from build123d import *

# Parameters (mm, degrees)
SKETCH_1_R      = 6.25
EXTRUDE_1_DEPTH = 15
SKETCH_2_W      = 27
SKETCH_2_H      = 18
EXTRUDE_2_DEPTH = 3
EXTRUDE_START   = 13.5
SKETCH_3_R      = 1.65
EXTRUDE_3_DEPTH = 5
EXTRUDE_START_2 = -13.5
SKETCH_3_2_R    = 1.65
EXTRUDE_4_DEPTH = 5
EXTRUDE_5_DEPTH = 5
SKETCH_5_R      = 2.5
EXTRUDE_6_DEPTH = 5


with BuildPart() as part:
    # ｽｹｯﾁ1 → ﾎﾞｽ - 押し出し1 (new body)
    with BuildSketch(Plane.XY):
        Circle(SKETCH_1_R)
    extrude(amount=EXTRUDE_1_DEPTH)

    # ｽｹｯﾁ2 → ﾎﾞｽ - 押し出し2 (add)
    with BuildSketch(Plane.XY.offset(15)):
        Rectangle(SKETCH_2_W, SKETCH_2_H)
    extrude(amount=EXTRUDE_2_DEPTH)

    # ｽｹｯﾁ3 → ﾎﾞｽ - 押し出し3 (add)
    with BuildSketch(Plane(origin=(0, 0, 0), x_dir=(0, 0, -1), z_dir=(1, 0, 0)).offset(EXTRUDE_START)):
        with BuildLine():
            Line((-18, 9), (-29.724032154, 4.69336906))
            ThreePointArc((-29.724032154, 4.69336906), (-33, 0), (-29.724032154, -4.69336906))
            Line((-29.724032154, -4.69336906), (-18, -9))
            Line((-18, -9), (-18, 9))
        make_face()
        with Locations((-28, 0)):
            Circle(SKETCH_3_R, mode=Mode.SUBTRACT)
    extrude(amount=-EXTRUDE_3_DEPTH)

    # ｽｹｯﾁ3<2> → ﾎﾞｽ - 押し出し4 (add)
    with BuildSketch(Plane(origin=(0, 0, 0), x_dir=(0, 0, -1), z_dir=(1, 0, 0)).offset(EXTRUDE_START_2)):
        with BuildLine():
            Line((-18, 9), (-29.724032154, 4.69336906))
            ThreePointArc((-29.724032154, 4.69336906), (-33, 0), (-29.724032154, -4.69336906))
            Line((-29.724032154, -4.69336906), (-18, -9))
            Line((-18, -9), (-18, 9))
        make_face()
        with Locations((-28, 0)):
            Circle(SKETCH_3_2_R, mode=Mode.SUBTRACT)
    extrude(amount=EXTRUDE_4_DEPTH)

    # ｽｹｯﾁ4 → ﾎﾞｽ - 押し出し5 (add, symmetric)
    with BuildSketch(Plane(origin=(0, 0, 0), x_dir=(1, 0, 0), z_dir=(0, 1, 0))):
        with BuildLine():
            Line((-13.5, -63), (-13.5, -3))
            ThreePointArc((-13.5, -3), (-43.5, -33), (-13.5, -63))
        make_face()
    extrude(amount=EXTRUDE_5_DEPTH, both=True)

    # ｽｹｯﾁ5 → ﾎﾞｽ - 押し出し6 (add)
    with BuildSketch(Plane.XY.offset(40)):
        with BuildLine():
            Line((-30, 5), (-30, 10))
            ThreePointArc((-30, 10), (-25, 15), (-20, 10))
            Line((-20, 10), (-20, 5))
            Line((-20, 5), (-30, 5))
        make_face()
        with Locations((-25, 10)):
            Circle(SKETCH_5_R, mode=Mode.SUBTRACT)
    extrude_6 = extrude(amount=EXTRUDE_6_DEPTH)

    # ﾐﾗｰ1: ﾎﾞｽ - 押し出し6 across plane
    add(extrude_6.mirror(Plane.ZX))


solid = part.part
Part model, mm, in its own coordinate system. A direction names the side the tool comes from. Give positions to 0.01 mm unless a question says otherwise; leave off trailing zeros. Loops run counter-clockwise (first coordinate to the right, second up) from the corner with the lowest first, then second, coordinate; pieces in that order, holes last.
(1) Pull direction X, two halves, no side cores. Call faces 6 (the cylindrical face through (-11.04, 0.07, 29.65)), 7 (the cylindrical face through (-25, 15, 42)), 8 (the cylindrical face through (-27, 8.5, 42.5)), 9 (the cylindrical face through (-27, -8.5, 42.5)): pulls with the +X half, pulls with the -X half, needs draft (parallel to the pull), parting line crosses it, or undercut.
Return value:
face 6: needs draft
face 7: parting line crosses it
face 8: undercut
face 9: undercut
(2) Band-saw the part on A-A (x = -10.5). Write the cut outline in (y, z).
Return value:
outline: (-9, 15) - (9, 15) - (9, 18) - (4.69, 29.72) arc R5 ccw to (-4.69, 29.72) - (-9, 18) - close; hole circle Ø3.3 at (0, 28)
(3) Band-saw the part on B-B (z = 25). Write the cut outline in (x, y), and give its area (3 significant figures).
Return value:
outline: (-42.41, -5) - (-13.5, -5) - (-13.5, -6.43) - (-8.5, -6.43) - (-8.5, 6.43) - (-13.5, 6.43) - (-13.5, 5) - (-42.41, 5) - close; (8.5, -6.43) - (13.5, -6.43) - (13.5, 6.43) - (8.5, 6.43) - close
area: 418 mm2
(4) Drill centre lines: line 1 along Y through (x, z) = (-25, 43.95); line 2 along X through (y, z) = (-10, 41.65); line 3 along Z through (x, y) = (-26.5, 6.5). Where is each one in solid material? Low to high.
Return value:
line 1: y = -15 to -12.5, -7.5 to 7.5, 12.5 to 15
line 2: x = -30 to -27.5, -22.5 to -20
line 3: z = 40 to 45
(5) 3-axis set-ups, long thin cutter, end or side, ignore diameter. For faces 1 (the flat face through (-13.5, 0, 9)), 2 (the flat face through (-20, 8, 42)), 3 (the flat face through (8.5, 0, 24)), 4 (the cylindrical face through (-11, 0, 33)), 5 (the flat face through (-13.5, 7, 20)): which of +Z, -Z, +X, -X, +Y, -Y reach the whole face in a straight line?
Return value:
face 1: -Z, +Y, -Y
face 2: +Z, -Z, +X, +Y
face 3: +Z, +Y, -Y
face 4: +Z, +X
face 5: +Z, -Z, -X, +Y
(6) Pin check, flat tips, straight feed: pin 1 (4 mm diameter, centred on y = -2.5, z = 22, fed in from -X); pin 2 (4 mm diameter, centred on y = 8, z = 43.5, fed in from -X); pin 3 (8.5 mm diameter, centred on x = -2.5, y = -2.5, fed in from +Z); pin 4 (4.5 mm diameter, centred on x = -25, y = -10, fed in from +Z). Stop position of each tip, or through.
Return value:
pin 1: stops at x = -42.12
pin 2: stops at x = -30
pin 3: stops at z = 18
pin 4: passes through
(7) Band-saw the part on D-D (x = -25). Write the cut outline in (y, z).
Return value:
outline: (-15, 40) - (-12.5, 40) - (-12.5, 45) - (-15, 45) - close; (-7.5, 40) - (-5, 40) - (-5, 5.29) - (5, 5.29) - (5, 40) - (7.5, 40) - (7.5, 45) - (5, 45) - (5, 60.71) - (-5, 60.71) - (-5, 45) - (-7.5, 45) - close; (12.5, 40) - (15, 40) - (15, 45) - (12.5, 45) - close
(8) Band-saw the part on C-C (y = 11). Write the cut outline in (x, z).
Return value:
outline: (-29.9, 40) - (-27.29, 40) - (-27.29, 45) - (-29.9, 45) - close; (-22.71, 40) - (-20.1, 40) - (-20.1, 45) - (-22.71, 45) - close
